Autodesk Fusion 360 part; units mm, degrees
sketch "Sketch1" plane through (0, 0, 0) normal (0, 0, 1) x (1, 0, 0)
  line L0 (31.5, -2) -> (-31.5, -2)
  line L1 (-31.5, -2) -> (-31.5, 2)
  line L2 (-31.5, 2) -> (31.5, 2)
  line L3 (31.5, 2) -> (31.5, -2)
  line L4 (31.5, -2) -> (-31.5, 2) construction
  line L5 (-31.5, -2) -> (31.5, 2) construction
  dimension "d8" = 4
  dimension "d9" = 63
extrude "Extrude1" add sketch "Sketch1" along normal mid plane 20 makes body 1
sketch "Sketch2" plane through (0, 0, 0) normal (0, 1, 0) x (1, 0, 0)
  arc A0 (25.0416, 2.5736) -> (-25.0416, 2.5736) centre (0, -39.2308) ccw
  arc A1 (-25.0416, -2.5736) -> (25.0416, -2.5736) centre (0, 39.2308) ccw
  circle A2 centre (-23.5, 0) radius 3
  circle A3 centre (23.5, 0) radius 3
  point P0 (-26.5, 0)
  point P1 (26.5, 0)
  point P2 (0, 9.5)
  point P3 (0, -9.5)
  dimension "d12" = 6
  dimension "d13" = 6
  dimension "d14" = 53
  dimension "d15" = 19
extrude "Extrude2" add sketch "Sketch2" along normal mid plane 4 separate body makes body 2
fillet "Fillet1" radius 1 8 edges at (0, 2, -9.5) (-26.5, 2, 0) (0, 2, 9.5) (26.5, 2, 0) (0, -2, -9.5) (26.5, -2, 0) (0, -2, 9.5) (-26.5, -2, 0) on bodies 2
sketch "Sketch4" plane through (0, 0, 0) normal (0, 0, 1) x (1, 0, 0)
hidden bodies 1
equation "LamelloLength = 53 mm"
equation "LamelloWidth = 19 mm"
equation "LamelloThickness = 4 mm"
equation "Tolerance = 1 mm"
equation "GrooveLength = LamelloLength + Tolerance + 9 mm"
equation "GrooveWidth = LamelloWidth + 1 mm"
equation "GrooveThickness = LamelloThickness"
equation "d8 = GrooveThickness"
equation "d9 = GrooveLength"
equation "d10 = GrooveWidth"
equation "d14 = LamelloLength"
equation "d15 = LamelloWidth"
equation "d16 = LamelloThickness"
properties part number "S10"
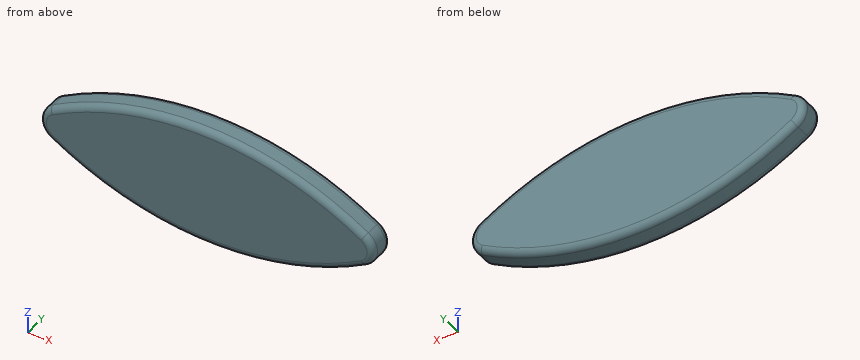
Work out the finished part from the listing and answer in its coordinate system (mm). Give positions to 0.01 mm unless a question says otherwise; leave off trailing zeros. Write each loop counter-clockwise with the first axis right and the second up, starting at its lowest first coordinate (ties: lowest second). Pieces come first, ordered by that corner, then holes. Notation, with made-up numbers: (47, 81.25) - (82, 81.25) arc R20 cw to (82, 86.25) - close; hole circle Ø2 at (-39, -38). An arc over 180 degrees is marked (long way). One line per item, written item: value. Start each with the question number.
1. Find section A-A (y = 0.1). Write down the section's boundary in (x, z).
2. Consider probe 1 along X at (y, z) = (-0.7, -0.25); probe 2 along Z at (x, y) = (-8.5, 0.05); probe 3 along Z at (x, y) = (23, 0). Determine where each line is inside the solid, lowest interval first.
3. Given pin 1 (2 mm diameter, centred on y = 1, z = 4, fed in from +X); pin 2 (2 mm diameter, centred on x = 17, y = 1, fed in from -Z), each flat-ended and moving along its own axis, determine where each tip first touches the part or whether it passes through.
Geometry results:
1. outline: (-25.04, -2.57) arc R48.73 ccw to (25.04, -2.57) arc R3 ccw to (25.04, 2.57) arc R48.73 ccw to (-25.04, 2.57) arc R3 ccw to start
2. probe 1: -26.49 to 26.49
2. probe 2: -8.75 to 8.75
2. probe 3: -3.73 to 3.73
3. pin 1: x = 24.32
3. pin 2: z = -6.8
